Autodesk Inventor part; units mm, degrees
ref_plane "YZ Plane" through (0, 0, 0) normal (1, 0, 0) x (0, 1, 0)
ref_plane "XZ Plane" through (0, 0, 0) normal (0, 1, 0) x (-1, 0, 0)
ref_plane "XY Plane" through (0, 0, 0) normal (0, 0, 1) x (1, 0, 0)
sketch "Sketch1" plane through (0, 0, 0) normal (0, 1, 0) x (-1, 0, 0)
  line L0 (0, 0) -> (50.8, 0)
  line L1 (50.8, 0) -> (50.8, -25.4)
  line L2 (50.8, -25.4) -> (0, -25.4)
  line L3 (0, -25.4) -> (0, 0)
  line L4 (47.625, -3.1826) -> (3.175, -3.1826)
  line L5 (3.175, -3.1826) -> (3.175, -22.225)
  line L6 (3.175, -22.225) -> (47.625, -22.225)
  line L7 (47.625, -22.225) -> (47.625, -3.1826)
  dimension "d0" = 50.8
  dimension "d1" = 25.4
  dimension "d2" = 3.175
  dimension "d3" = 3.1826
  dimension "d4" = 3.175
  dimension "d5" = 3.175
extrude "Extrusion1" add sketch "Sketch1" along normal blind 304.8
sketch "Sketch2" plane through (0, 0, 0) normal (1, 0, 0) x (0, 0, -1)
  line L0 (25.4, 0) -> (25.4, 304.8)
  line L1 (0, 304.8) -> (25.4, 304.8)
  line L2 (25.4, 304.8) -> (25.4, 254)
  line L3 (25.4, 254) -> (0, 254)
  line L4 (0, 254) -> (0, 304.8)
  line L5 (3.1826, 0) -> (3.1826, 304.8)
  line L6 (3.1826, 301.7936) -> (22.225, 301.7936)
  line L7 (22.225, 301.7936) -> (22.225, 257.175)
  line L8 (22.225, 257.175) -> (3.1826, 257.175)
  line L9 (3.1826, 257.175) -> (3.1826, 301.7936)
  point P0 (0, 0)
  dimension "d8" = 50.8
  dimension "d9" = 3.175
  dimension "d10" = 3.175
extrude "Extrusion2" add sketch "Sketch2" along normal blind 50.8 contours L3 L5 L8 L7 L6 L1 L0 | L3 L4 L1 L5
sketch "Sketch3" plane through (0, 0, -25.4) normal (0, 0, -1) x (-1, 0, 0)
  circle A0 centre (-25.4, 280.6907) radius 14.2875
  line L0 (-50.8, 254) -> (-50.8, 304.8)
  point P0 (0, 0)
  dimension "d13" = 25.4
  dimension "d14" = 28.575
extrude "Extrusion3" cut sketch "Sketch3" against normal through all
sketch "Sketch4" plane through (0, 0, -25.4) normal (0, 0, -1) x (-1, 0, 0)
  circle A0 centre (24.6023, 25.4) radius 14.2875
  line L0 (50.8, 0) -> (0, 0)
  dimension "d17" = 25.4
  dimension "d18" = 28.575
extrude "Extrusion4" cut sketch "Sketch4" against normal through all
sketch "Sketch5" plane through (0, 0, -25.4) normal (0, 0, -1) x (-1, 0, 0)
  circle A0 centre (25.4, 279.4) radius 14.2875
  line L0 (50.8, 304.8) -> (-50.8, 304.8)
  line L1 (50.8, 0) -> (50.8, 304.8)
  point P0 (0, 0)
  dimension "d21" = 25.4
  dimension "d22" = 28.575
  dimension "d23" = 25.4
extrude "Extrusion5" cut sketch "Sketch5" against normal blind 25.4
properties part number "arm" material "Aluminum 6061"
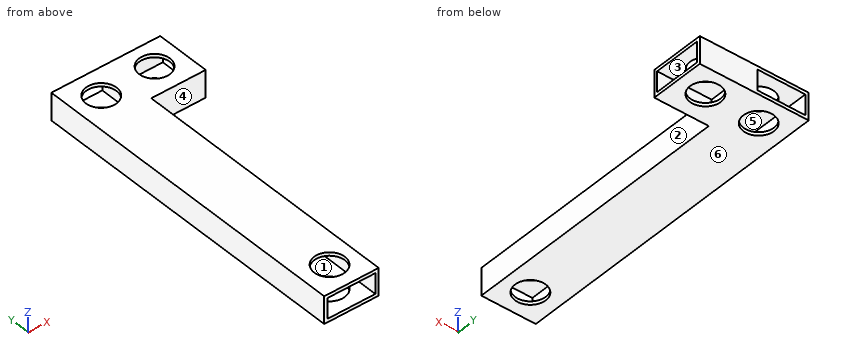
The listing builds one solid part. Answer for the finished solid, in the listing's coordinates (mm). Face numbers are marked on the shaded views. A direction names the side the tool comes from. Coordinates: 2 decimals unless noted, no trailing zeros. Order: outer loops, then holes, each group sorted by start corner. A loop starts at its lowest first (then second) coordinate and runs counter-clockwise, first axis right, second up.
Q1. A cutting plane is placed at C-C, the plane z = -13. Write down the section's boundary in (x, y) (3 decimals), and give its area (3 significant figures).
Q2. Which of the six approach directions +Z, -Z, +X, -X, +Y, -Y give full straight-line access (tool end or side, diameter ignored) to the marked faces 1, 2 and 3?
Q3. A cutting plane is placed at B-B, the plane y = 90.5. Write down the section's boundary in (x, z) (3 decimals).
Q4. A cutting plane is placed at D-D, the plane x = -25.5. Write down the section's boundary in (y, z) (3 decimals).
Q5. Consider line 1 (Y direction, x = -25.4, z = -2.15); line 2 (X direction, y = 173, z = -11) (3 decimals); line 3 (Z direction, x = -40, y = 233) (3 decimals). Determine where each line is inside the solid, lowest interval first.
Q6. For a pull along Z with two mould halves and no side action, classify the marked faces 4, 5 and 6 as pulls with the +Z half, pulls with the -Z half, needs draft (parallel to the pull), parting line crosses it, or undercut.
Q7. Given P1, Ø1, axis at y = 149.5, z = -14.5, coming from the +X side; P2, Ø12.5, axis at x = 28, z = -9, coming from the -Y side, each flat-ended and moving along its own axis, determine where each tip first touches the part or whether it passes through.
Q8. A cutting plane is placed at A-A, the plane x = -7. Write down the section's boundary in (y, z) (3 decimals).
Answers follow:
1. outline: (-50.8, 0) - (-47.625, 0) - (-47.625, 304.8) - (-50.8, 304.8) - close; (-3.175, 0) - (0, 0) - (0, 254) - (50.8, 254) - (50.8, 257.175) - (0, 257.175) - (0, 301.794) - (50.8, 301.794) - (50.8, 304.8) - (-3.175, 304.8) - close
1. area: 2,250 mm2
2. face 1: +Y, -Y
2. face 2: +Z, -Z, +X, -Y
2. face 3: +X
3. outline: (-50.8, -25.4) - (0, -25.4) - (0, 0) - (-50.8, 0) - close; hole (-47.625, -22.225) - (-3.175, -22.225) - (-3.175, -3.183) - (-47.625, -3.183) - close
4. outline: (0, -25.4) - (11.141, -25.4) - (11.141, -22.225) - (0, -22.225) - close; (0, -3.183) - (11.141, -3.183) - (11.141, 0) - (0, 0) - close; (39.659, -25.4) - (265.113, -25.4) - (265.113, -22.225) - (39.659, -22.225) - close; (39.659, -3.183) - (265.113, -3.183) - (265.113, 0) - (39.659, 0) - close; (293.687, -25.4) - (304.8, -25.4) - (304.8, -22.225) - (293.687, -22.225) - close; (293.687, -3.183) - (304.8, -3.183) - (304.8, 0) - (293.687, 0) - close
5. line 1: y = 0 to 11.13, 39.67 to 265.11, 293.69 to 304.8
5. line 2: x = -50.8 to -47.625, -3.175 to 0
5. line 3: z = -25.4 to -22.225, -3.183 to 0
6. face 4: needs draft
6. face 5: undercut
6. face 6: pulls with the -Z half
7. P1: stops at x = 0
7. P2: stops at y = 254
8. outline: (0, -25.4) - (304.8, -25.4) - (304.8, -22.225) - (0, -22.225) - close; (0, -3.183) - (304.8, -3.183) - (304.8, 0) - (0, 0) - close
